from build123d import *

# Parameters (mm, degrees)
F0_R     = 10.5
F0_R_2   = 9.5
F1_DEPTH = 40
F2_W     = 5
F2_H     = 2
F3_DEPTH = 40.001


with BuildPart() as f1:
    # F0 (on Top) → F1 (new body)
    with BuildSketch(Plane.XY):
        with Locations((-88.5, -95)):
            Circle(F0_R)
        with Locations((-88.5, -95)):
            Circle(F0_R_2, mode=Mode.SUBTRACT)
    extrude(amount=F1_DEPTH)

    # F2 (on face) → F3 (cut, through all)
    with BuildSketch(Plane.XY.offset(40)):
        with Locations((-100.125511, -95)):
            Rectangle(F2_W, F2_H)
    extrude(amount=-F3_DEPTH, mode=Mode.SUBTRACT)


with BuildPart() as f1_1:
    # F4: moved
    add(f1.part.moved(Location((0, 0, 50))))


solid = f1_1.part
Input: part model. Units: mm. Frame: model coordinates. A direction names the side the tool comes from. Give positions to 0.01 mm unless a question says otherwise; leave off trailing zeros. Write each loop counter-clockwise with the first axis right and the second up, starting at its lowest first coordinate (ties: lowest second). Pieces come first, ordered by that corner, then holes.
Q1. Set-up query: faces 3 (the face through (-98.5, -96, 70.3)), 4 (the face through (-83, -87, 50)). Return all of +Z, -Z, +X, -X, +Y, -Y with unobstructed straight access to the full face (end or side cutting, diameter ignored); none if empty.
Q2. Section C-C, the plane x = -92.25. Output: boundary loops of the cut face in (y, z), plus the area to 3 significant figures.
Q3. Section A-A, the plane x = -82.75. Output: boundary loops of the cut face in (y, z).
Q4. Section B-B, the plane z = 53. Output: boundary loops of the cut face in (x, y), plus the area to 3 significant figures.
Q5. First-contact query: P1, Ø10, axis at y = -103, z = 76.5, coming from the +X side; P2, Ø8, axis at x = -82.5, z = 85.5, coming from the +Y side; P3, Ø4, axis at x = -84, z = 63, coming from the +Y side; P4, Ø2, axis at x = -96.5, y = -103.5, coming from the +Z side. Flat tips, straight axial feed; report the tip coordinate or a pass-through.
Q6. Pull-direction query (Y, two-part tool) for faces 1 (the face through (-83, -87, 90)), 2 (the face through (-98.5, -94, 70.3)); classes: pulls with the +Y half, pulls with the -Y half, needs draft (parallel to the pull), parting line crosses it, or undercut.
Q7. Material intervals for probe 1 along Y at (x, z) = (-89.75, 76.5); probe 2 along X at (y, z) = (-90, 76.5); probe 3 along Y at (x, z) = (-92, 61), sorted ascending.
Filled in:
1. face 3: +Z, -Z, -X
1. face 4: -Z, +X, -X, +Y, -Y
2. outline: (-104.81, 50) - (-103.73, 50) - (-103.73, 90) - (-104.81, 90) - close; (-86.27, 50) - (-85.19, 50) - (-85.19, 90) - (-86.27, 90) - close
2. area: 86.3 mm2
3. outline: (-103.79, 50) - (-102.56, 50) - (-102.56, 90) - (-103.79, 90) - close; (-87.44, 50) - (-86.21, 50) - (-86.21, 90) - (-87.44, 90) - close
4. outline: (-98.95, -96) arc R10.5 ccw (long way) to (-98.95, -94) - (-97.95, -94) arc R9.5 cw (long way) to (-97.95, -96) - close
4. area: 60.8 mm2
5. P1: stops at x = -78.44
5. P2: stops at y = -84.69
5. P3: stops at y = -84.8
5. P4: passes through
6. face 1: needs draft
6. face 2: undercut
7. probe 1: y = -105.43 to -104.42, -85.58 to -84.57
7. probe 2: x = -97.73 to -96.58, -80.42 to -79.27
7. probe 3: y = -104.9 to -103.83, -86.17 to -85.1
